from build123d import *

# Parameters (mm, degrees)
SKETCH_1_W          = 10.2
SKETCH_1_H          = 5
EXTRUDE_1_DEPTH     = 2.8
SKETCH_2_R          = 1
EXTRUDE_2_DEPTH     = 0.5
SKETCH_3_R          = 0.4
EXTRUDE_3_DEPTH     = 1
SKETCH_4_R          = 0.7
EXTRUDE_4_DEPTH     = 5.8
SKETCH_5_R          = 0.6
CUT_EXTRUDE_1_DEPTH = 0.25
FILLET_1_R          = 0.6
FILLET_2_R          = 0.2


with BuildPart() as part:
    # 草图1 → 凸台-拉伸1 (new body)
    with BuildSketch(Plane(origin=(0, 0, 0), x_dir=(1, 0, 0), z_dir=(0, 1, 0))):
        with Locations((5.1, 2.5)):
            Rectangle(SKETCH_1_W, SKETCH_1_H)
    extrude(amount=EXTRUDE_1_DEPTH)

    # 草图2 → 凸台-拉伸2 (add)
    with BuildSketch(Plane(origin=(0, 2.8, 0), x_dir=(1, 0, 0), z_dir=(0, 1, 0))):
        with Locations(Location((1.29, 3.77, 0), (0, 0, 90))):
            Circle(SKETCH_2_R)
        with Locations(Location((3.83, 3.77, 0), (0, 0, 90))):
            Circle(SKETCH_2_R)
        with Locations(Location((6.37, 3.77, 0), (0, 0, 90))):
            Circle(SKETCH_2_R)
        with Locations(Location((8.91, 3.77, 0), (0, 0, 90))):
            Circle(SKETCH_2_R)
        with Locations(Location((3.83, 1.23, 0), (0, 0, 90))):
            Circle(SKETCH_2_R)
        with Locations(Location((6.37, 1.23, 0), (0, 0, 90))):
            Circle(SKETCH_2_R)
        with Locations(Location((8.91, 1.23, 0), (0, 0, 90))):
            Circle(SKETCH_2_R)
        with Locations(Location((1.29, 1.23, 0), (0, 0, 90))):
            Circle(SKETCH_2_R)
    extrude(amount=EXTRUDE_2_DEPTH)

    # 草图3 → 凸台-拉伸3 (add)
    with BuildSketch(Plane(origin=(0, 3.3, 0), x_dir=(1, 0, 0), z_dir=(0, 1, 0))):
        with Locations(Location((1.29, 1.23, 0), (0, 0, 270))):
            Circle(SKETCH_3_R)
        with Locations(Location((3.83, 1.23, 0), (0, 0, 270))):
            Circle(SKETCH_3_R)
        with Locations(Location((6.37, 1.23, 0), (0, 0, 270))):
            Circle(SKETCH_3_R)
        with Locations(Location((8.91, 1.23, 0), (0, 0, 270))):
            Circle(SKETCH_3_R)
        with Locations(Location((3.83, 3.77, 0), (0, 0, 270))):
            Circle(SKETCH_3_R)
        with Locations(Location((6.37, 3.77, 0), (0, 0, 270))):
            Circle(SKETCH_3_R)
        with Locations(Location((8.91, 3.77, 0), (0, 0, 270))):
            Circle(SKETCH_3_R)
        with Locations(Location((1.29, 3.77, 0), (0, 0, 270))):
            Circle(SKETCH_3_R)
    extrude(amount=EXTRUDE_3_DEPTH)

    # 草图4 → 凸台-拉伸4 (add)
    with BuildSketch(Plane(origin=(0, 3.3, 0), x_dir=(1, 0, 0), z_dir=(0, 1, 0))):
        with Locations(Location((1.29, 1.23, 0), (0, 0, 270))):
            Circle(SKETCH_4_R)
        with Locations(Location((3.83, 1.23, 0), (0, 0, 270))):
            Circle(SKETCH_4_R)
        with Locations(Location((6.37, 1.23, 0), (0, 0, 270))):
            Circle(SKETCH_4_R)
        with Locations(Location((8.91, 1.23, 0), (0, 0, 270))):
            Circle(SKETCH_4_R)
        with Locations(Location((3.83, 3.77, 0), (0, 0, 270))):
            Circle(SKETCH_4_R)
        with Locations(Location((6.37, 3.77, 0), (0, 0, 270))):
            Circle(SKETCH_4_R)
        with Locations(Location((8.91, 3.77, 0), (0, 0, 270))):
            Circle(SKETCH_4_R)
        with Locations(Location((1.29, 3.77, 0), (0, 0, 270))):
            Circle(SKETCH_4_R)
    extrude(amount=-EXTRUDE_4_DEPTH)

    # 草图5 → 切除-拉伸1 (cut)
    with BuildSketch(Plane.XZ.offset(2.5)):
        with Locations(Location((8.91, -1.23, 0), (0, 0, 270))):
            Circle(SKETCH_5_R)
        with Locations(Location((6.37, -1.23, 0), (0, 0, 270))):
            Circle(SKETCH_5_R)
        with Locations(Location((3.83, -1.23, 0), (0, 0, 270))):
            Circle(SKETCH_5_R)
        with Locations(Location((1.29, -1.23, 0), (0, 0, 270))):
            Circle(SKETCH_5_R)
        with Locations(Location((6.37, -3.77, 0), (0, 0, 270))):
            Circle(SKETCH_5_R)
        with Locations(Location((3.83, -3.77, 0), (0, 0, 270))):
            Circle(SKETCH_5_R)
        with Locations(Location((1.29, -3.77, 0), (0, 0, 270))):
            Circle(SKETCH_5_R)
        with Locations(Location((8.91, -3.77, 0), (0, 0, 270))):
            Circle(SKETCH_5_R)
    extrude(amount=-CUT_EXTRUDE_1_DEPTH, mode=Mode.SUBTRACT)

    # 圆角1
    # the kernel refuses this fillet: 0.6 mm, written as the material it adds along each edge
    with BuildSketch(Plane(origin=(6.37, -2.25, -3.77), x_dir=(0, 0, -1), z_dir=(-1, 0, 0))) as fillet_1_piece_1:
        with BuildLine():
            CenterArc((0.112660283, 0.6), FILLET_1_R, 270, 54.314665288)
            Line((0.112660283, 0), (0.112660283, -0.012))
            Line((0.112660283, -0.012), (0.6, -0.012))
            Line((0.6, -0.012), (0.612, 0))
            ThreePointArc((0.612, 0), (0.612, 0.125), (0.609746794, 0.243))
            Line((0.609746794, 0.243), (0.6, 0.25))
        make_face()
    revolve(axis=Axis((6.37, -2.25, -3.77), (0, -1, 0)))
    with BuildSketch(Plane(origin=(1.29, -2.25, -1.23), x_dir=(0, 0, -1), z_dir=(-1, 0, 0))) as fillet_1_piece_2:
        with BuildLine():
            CenterArc((0.112660283, 0.6), FILLET_1_R, 270, 54.314665288)
            Line((0.112660283, 0), (0.112660283, -0.012))
            Line((0.112660283, -0.012), (0.6, -0.012))
            Line((0.6, -0.012), (0.612, 0))
            ThreePointArc((0.612, 0), (0.612, 0.125), (0.609746794, 0.243))
            Line((0.609746794, 0.243), (0.6, 0.25))
        make_face()
    revolve(axis=Axis((1.29, -2.25, -1.23), (0, -1, 0)))
    with BuildSketch(Plane(origin=(3.83, -2.25, -1.23), x_dir=(0, 0, -1), z_dir=(-1, 0, 0))) as fillet_1_piece_3:
        with BuildLine():
            CenterArc((0.112660283, 0.6), FILLET_1_R, 270, 54.314665288)
            Line((0.112660283, 0), (0.112660283, -0.012))
            Line((0.112660283, -0.012), (0.6, -0.012))
            Line((0.6, -0.012), (0.612, 0))
            ThreePointArc((0.612, 0), (0.612, 0.125), (0.609746794, 0.243))
            Line((0.609746794, 0.243), (0.6, 0.25))
        make_face()
    revolve(axis=Axis((3.83, -2.25, -1.23), (0, -1, 0)))
    with BuildSketch(Plane(origin=(6.37, -2.25, -1.23), x_dir=(0, 0, -1), z_dir=(-1, 0, 0))) as fillet_1_piece_4:
        with BuildLine():
            CenterArc((0.112660283, 0.6), FILLET_1_R, 270, 54.314665288)
            Line((0.112660283, 0), (0.112660283, -0.012))
            Line((0.112660283, -0.012), (0.6, -0.012))
            Line((0.6, -0.012), (0.612, 0))
            ThreePointArc((0.612, 0), (0.612, 0.125), (0.609746794, 0.243))
            Line((0.609746794, 0.243), (0.6, 0.25))
        make_face()
    revolve(axis=Axis((6.37, -2.25, -1.23), (0, -1, 0)))
    with BuildSketch(Plane(origin=(3.83, -2.25, -3.77), x_dir=(0, 0, -1), z_dir=(-1, 0, 0))) as fillet_1_piece_5:
        with BuildLine():
            CenterArc((0.112660283, 0.6), FILLET_1_R, 270, 54.314665288)
            Line((0.112660283, 0), (0.112660283, -0.012))
            Line((0.112660283, -0.012), (0.6, -0.012))
            Line((0.6, -0.012), (0.612, 0))
            ThreePointArc((0.612, 0), (0.612, 0.125), (0.609746794, 0.243))
            Line((0.609746794, 0.243), (0.6, 0.25))
        make_face()
    revolve(axis=Axis((3.83, -2.25, -3.77), (0, -1, 0)))
    with BuildSketch(Plane(origin=(1.29, -2.25, -3.77), x_dir=(0, 0, -1), z_dir=(-1, 0, 0))) as fillet_1_piece_6:
        with BuildLine():
            CenterArc((0.112660283, 0.6), FILLET_1_R, 270, 54.314665288)
            Line((0.112660283, 0), (0.112660283, -0.012))
            Line((0.112660283, -0.012), (0.6, -0.012))
            Line((0.6, -0.012), (0.612, 0))
            ThreePointArc((0.612, 0), (0.612, 0.125), (0.609746794, 0.243))
            Line((0.609746794, 0.243), (0.6, 0.25))
        make_face()
    revolve(axis=Axis((1.29, -2.25, -3.77), (0, -1, 0)))
    with BuildSketch(Plane(origin=(8.91, -2.25, -3.77), x_dir=(0, 0, -1), z_dir=(-1, 0, 0))) as fillet_1_piece_7:
        with BuildLine():
            CenterArc((0.112660283, 0.6), FILLET_1_R, 270, 54.314665288)
            Line((0.112660283, 0), (0.112660283, -0.012))
            Line((0.112660283, -0.012), (0.6, -0.012))
            Line((0.6, -0.012), (0.612, 0))
            ThreePointArc((0.612, 0), (0.612, 0.125), (0.609746794, 0.243))
            Line((0.609746794, 0.243), (0.6, 0.25))
        make_face()
    revolve(axis=Axis((8.91, -2.25, -3.77), (0, -1, 0)))
    with BuildSketch(Plane(origin=(8.91, -2.25, -1.23), x_dir=(0, 0, -1), z_dir=(-1, 0, 0))) as fillet_1_piece_8:
        with BuildLine():
            CenterArc((0.112660283, 0.6), FILLET_1_R, 270, 54.314665288)
            Line((0.112660283, 0), (0.112660283, -0.012))
            Line((0.112660283, -0.012), (0.6, -0.012))
            Line((0.6, -0.012), (0.612, 0))
            ThreePointArc((0.612, 0), (0.612, 0.125), (0.609746794, 0.243))
            Line((0.609746794, 0.243), (0.6, 0.25))
        make_face()
    revolve(axis=Axis((8.91, -2.25, -1.23), (0, -1, 0)))

    # 圆角2
    fillet_2_edges = [part.edges().sort_by_distance(p)[0] for p in [
        (0, 1.4, -5),
        (10.2, 1.4, -5),
        (10.2, 1.4, 0),
        (0, 1.4, 0),
    ]]
    fillet(fillet_2_edges, radius=FILLET_2_R)


solid = part.part
Can you work these out from the model? Positions are in its coordinate system, mm. A direction names the side the tool comes from. Give positions to 0.01 mm unless a question says otherwise; leave off trailing zeros. Loops run counter-clockwise (first coordinate to the right, second up) from the corner with the lowest first, then second, coordinate; pieces in that order, holes last. Notation, with made-up numbers: M -0.75,40.25 L 18.25,40.25 A27 cw 18.25,70.25 Z; hole C -4.5,77.25 d2. An arc over 180 degrees is marked long. One line per item, written item: value. Start each with the question number.
1) If I drill on line 1 (Z direction, x = 1.25, y = 3.5); line 2 (X direction, y = -1.25, z = -4.2); line 3 (Y direction, x = 3, z = -2.5), over which ranges is the centre line in solid material (lowest first)? Write a range as [from, to].
2) If we section it at D-D, the plane z = -2.5: Write out the boundary of the cut face in (x, y), and give its area (3 significant figures).
3) If we section it at A-A, the plane y = 3.5: Write out the boundary of the cut face in (x, z), and give its area (3 significant figures).
4) If we section it at B-B, the plane y = -1.5: Write out the boundary of the cut face in (x, z), and give its area (3 significant figures).
5) If we section it at C-C, the plane x = 9.75: Write out the boundary of the cut face in (y, z), and give its area (3 significant figures).
6) On a 3-axis mill with a long thin cutter (end or side, diameter ignored), from which of +Z, -Z, +X, -X, +Y, -Y can I reach the whole of each face in a straight line? I mean faces 1 (the face through (4.42, -1.23, -0.85)), 2 (the face through (6.07, 3.046, -2.184)), 3 (the face through (5, 1, 0)). Say none if no direction works.
7) Thinking about a two-plate mould opening in X: for faces 4 (the face through (10.2, 1, -2)), 5 (the face through (2, 3.3, -4)), 6 (the face through (0, 1, -2)), 7 (the face through (8.07, 3.05, -4.31)), which applies, +X half, -X half, draft (parallel to the pull), parting line (faces both ways), or undercut?
Completed:
1. line 1: z = [-4.17, -3.37], [-1.63, -0.83]
1. line 2: x = [0.74, 1.84], [3.28, 4.38], [5.82, 6.92], [8.36, 9.46]
1. line 3: y = [0, 2.8]
2. outline: M 0,0 L 10.2,0 L 10.2,2.8 L 0,2.8 Z
2. area: 28.6 mm^2
3. outline: C 1.29,-3.77 d0.8; C 1.29,-1.23 d0.8; C 3.83,-3.77 d0.8; C 3.83,-1.23 d0.8; C 6.37,-3.77 d0.8; C 6.37,-1.23 d0.8; C 8.91,-3.77 d0.8; C 8.91,-1.23 d0.8
3. area: 4.02 mm^2
4. outline: C 1.29,-3.77 d1.4; C 1.29,-1.23 d1.4; C 3.83,-3.77 d1.4; C 3.83,-1.23 d1.4; C 6.37,-3.77 d1.4; C 6.37,-1.23 d1.4; C 8.91,-3.77 d1.4; C 8.91,-1.23 d1.4
4. area: 12.3 mm^2
5. outline: M 0,-5 L 2.8,-5 L 2.8,-4.31 L 3.3,-4.31 L 3.3,-3.23 L 2.8,-3.23 L 2.8,-1.77 L 3.3,-1.77 L 3.3,-0.69 L 2.8,-0.69 L 2.8,0 L 0,0 Z
5. area: 15.1 mm^2
6. face 1: -Y
6. face 2: +Y
6. face 3: +Z, +X, -X, +Y, -Y
7. face 4: +X half
7. face 5: undercut
7. face 6: -X half
7. face 7: undercut
